from build123d import *

# Parameters (mm, degrees)
CUT_EXTRUDE1_START = 14.7828
CUT_EXTRUDE1_DEPTH = 2.0828


with BuildPart() as part:
    # Sketch2 → Revolve1 (revolve)
    with BuildSketch(Plane(origin=(0, 0, 0), x_dir=(0, 0, -1), z_dir=(1, 0, 0)), mode=Mode.PRIVATE) as revolve1_sk:
        with BuildLine():
            Line((14.7828, 0), (14.7828, 1.60655))
            Line((14.7828, 1.60655), (14.30655, 2.0828))
            Line((14.30655, 2.0828), (-10.6172, 2.0828))
            Line((-10.6172, 2.0828), (-10.6172, 3.22072))
            ThreePointArc((-10.6172, 3.22072), (-10.6782038, 3.3679962), (-10.82548, 3.429))
            Line((-10.82548, 3.429), (-14.57452, 3.429))
            ThreePointArc((-14.57452, 3.429), (-14.7217962, 3.3679962), (-14.7828, 3.22072))
            Line((-14.7828, 3.22072), (-14.7828, 0))
            Line((-14.7828, 0), (14.7828, 0))
        make_face()
    revolve(revolve1_sk.sketch.rotate(Axis((0, 0, -14.7828), (0, 0, 1)), 90), axis=Axis((0, 0, -14.7828), (0, 0, 1)))

    # Sketch3 → Cut-Extrude1 (cut)
    with BuildSketch(Plane.XY.offset(CUT_EXTRUDE1_START)):
        Polygon((-1.7859375, 1.031111496), (-1.7859375, -1.031111496), (0, -2.062222993), (1.7859375, -1.031111496), (1.7859375, 1.031111496), (0, 2.062222993), align=None)
    extrude(amount=-CUT_EXTRUDE1_DEPTH, mode=Mode.SUBTRACT)

    # Cut-Extrude2 cone 1 section (through the dimple's axis) → Cut-Extrude2 (revolve, cut)
    with BuildSketch(Plane(origin=(0, 0, 14.7828), x_dir=(0, -1, 0), z_dir=(1, 0, 0))):
        Polygon((0, 0), (2.255305827, 0), (0, 1.302101426), align=None)
    revolve(axis=Axis((0, 0, 14.7828), (0, 0, -1)), mode=Mode.SUBTRACT)


solid = part.part
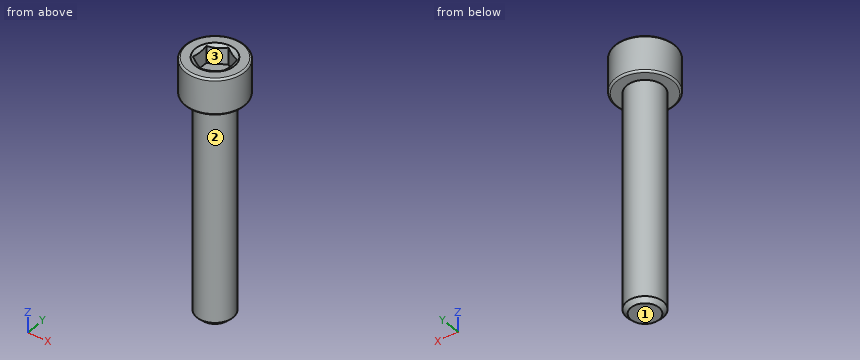
The model under review builds one solid part; all positions refer to its coordinate system, in mm. Face numbers are marked on the shaded views. Coordinates: 2 decimals unless noted, no trailing zeros. Order: outer loops, then holes, each group sorted by start corner. A loop starts at its lowest first (then second) coordinate and runs counter-clockwise, first axis right, second up. Notation, with made-up numbers: (89, 24.25) -> (116, 24.25) arc R28 ccw to (116, 57.25) -> close; hole circle Ø4 at (55, 19). An arc over 180 degrees is marked (long way). Answer in a Markdown table with one row per item.
(1) Wall thickness on line 1 along Z through (x, y) = (-0.75, 0); line 2 along Y through (x, z) = (1.75, 13); line 3 along Z through (x, y) = (2, 2): over which ranges is each line inside the solid? List them lowest first.
Answers:
| item | result |
|---|---|
| line 1 | -14.78 to 12.7 |
| line 2 | -2.95 to -1.05, 1.05 to 2.95 |
| line 3 | 10.62 to 14.78 |
(2) The part is to be moulded in two halves that separate along Y. For the marked faces 1, 2 and 3, say which applies: +Y half, -Y half, draft (parallel to the pull), parting line (faces both ways), or undercut.
Answers:
| item | result |
|---|---|
| face 1 | draft |
| face 2 | parting line |
| face 3 | undercut |
(3) Consider section A-A (z = -1.75). Write out the cut boundary in (x, y).
Answers:
| item | result |
|---|---|
| outline | circle Ø4.17 at (0, 0) |
(4) Insertion check: pin 1 (1.8 mm diameter, centred on x = -0.5, y = 0, fed in from +Z); pin 2 (3 mm diameter, centred on y = -0.5, z = -4.5, fed in from -X). Each pin has a flat end and moves straight along its axis. Give the tip position at first contact, or say it passes through.
Answers:
| item | result |
|---|---|
| pin 1 | z = 12.7 |
| pin 2 | x = -2.08 |
